Answer from the drawing. Dimensions are ordinates in mm from the lowest x, y and z of the part. A direction names the side the tool comes from. Round coordinates to 2 decimals unless told otherwise and drop trailing zeros. Loops run counter-clockwise (first coordinate to the right, second up) from the corner with the lowest first, then second, coordinate; pieces in that order, holes last. Notation, with made-up numbers: (84.25, 56) - (96.25, 56) arc R16 ccw to (96.25, 68) - close; hole circle Ø8 at (42.25, 39). An arc over 180 degrees is marked (long way). Write item = value, one per line. Start each with the question number.
1) Section B-B, the plane z = 3.75 is taken. Determine the outline of the cut face in (x, y).
2) Straight lines are drawn through the part: line 1 along Y through (x, z) = (8.75, 6); line 2 along X through (y, z) = (0.8, 2.25); line 3 along Y through (x, z) = (5.25, 8). For each, find the intervals that lie inside material, in ascending order.
3) Given pin 1 Ø1 at (x, y) = (7, 1) entering from +Z; pin 2 Ø4 at (x, z) = (4.5, 4.5) entering from -Y, each flat-ended and moving along its own axis, determine where each tip first touches the part or whether it passes through.
4) Section A-A, the plane y = 1.25 is taken. Determine the outline of the cut face in (x, z).
5) Section C-C, the plane x = 7.75 is taken. Determine the outline of the cut face in (y, z), and give its area (3 significant figures).
6) A tool of negligible diameter and unlimited length cuts with its end or side. For the marked faces 1 and 2, from which of +Z, -Z, +X, -X, +Y, -Y can it reach the whole face along a straight path? Write none if from no direction.
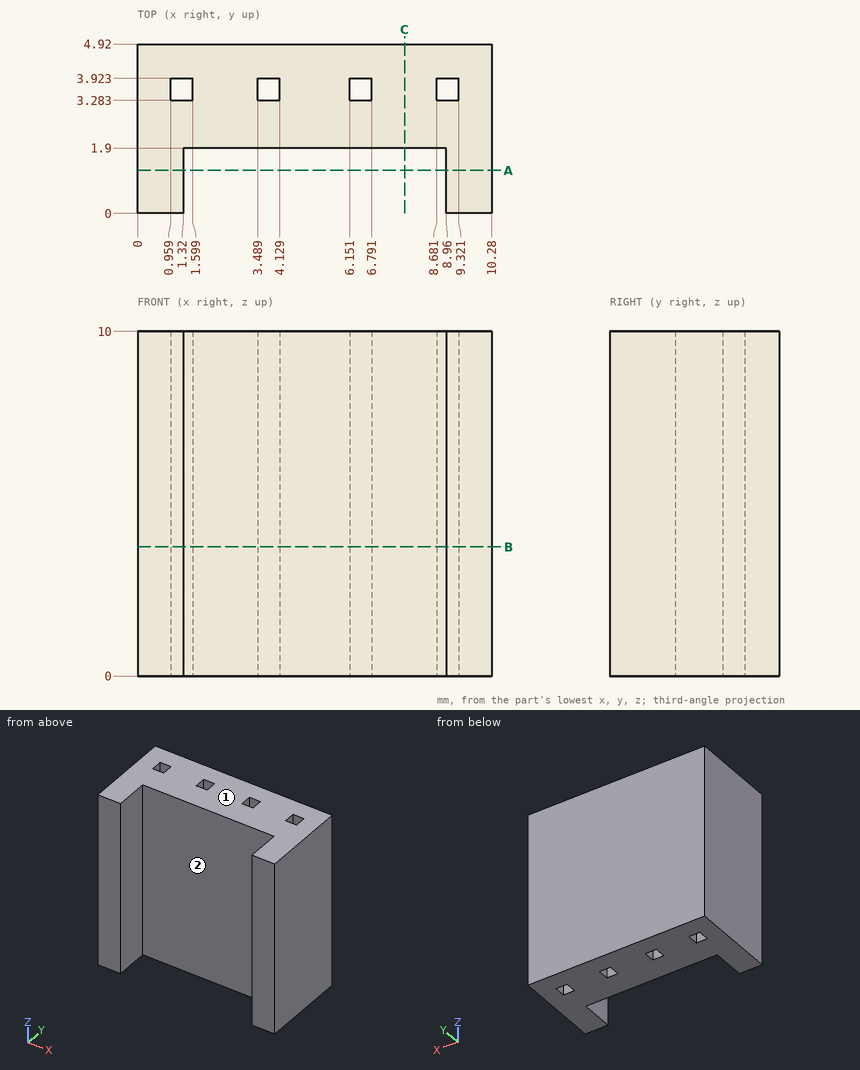
Geometry check:
q1.outline = (0, 0) - (1.32, 0) - (1.32, 1.9) - (8.96, 1.9) - (8.96, 0) - (10.28, 0) - (10.28, 4.92) - (0, 4.92) - close; hole (0.96, 3.28) - (1.6, 3.28) - (1.6, 3.92) - (0.96, 3.92) - close; hole (3.49, 3.28) - (4.13, 3.28) - (4.13, 3.92) - (3.49, 3.92) - close; hole (6.15, 3.28) - (6.79, 3.28) - (6.79, 3.92) - (6.15, 3.92) - close; hole (8.68, 3.28) - (9.32, 3.28) - (9.32, 3.92) - (8.68, 3.92) - close
q2.line_1 = 1.9 to 3.28, 3.92 to 4.92
q2.line_2 = 0 to 1.32, 8.96 to 10.28
q2.line_3 = 1.9 to 4.92
q3.pin_1 = through
q3.pin_2 = 1.9
q4.outline = (0, 0) - (1.32, 0) - (1.32, 10) - (0, 10) - close; (8.96, 0) - (10.28, 0) - (10.28, 10) - (8.96, 10) - close
q5.outline = (1.9, 0) - (4.92, 0) - (4.92, 10) - (1.9, 10) - close
q5.area = 30.2 mm2
q6.face_1 = +Z, +X, -X, +Y, -Y
q6.face_2 = +Z, -Z, -Y
